from build123d import *

# Parameters (mm, degrees)
F0_W     = 622.3
F0_H     = 530.225
F0_R     = 2.413
F0_R_2   = 4.7625
F0_W_2   = 210.82
F0_H_2   = 310.388
F1_DEPTH = 25.4
F2_T     = -2.54
F3_W     = 617.22
F3_H     = 22.86
F4_DEPTH = 525.145


with BuildPart() as f1:
    # F0 (on Front) → F1 (new body)
    with BuildSketch(Plane.XZ):
        with Locations((0, 265.1125)):
            Rectangle(F0_W, F0_H)
        with Locations((-190.5, 54.483)):
            Circle(F0_R, mode=Mode.SUBTRACT)
        with Locations((-292.1, 95.25)):
            Circle(F0_R_2, mode=Mode.SUBTRACT)
        with Locations((-259.588, 91.694)):
            Circle(F0_R, mode=Mode.SUBTRACT)
        with Locations((-88.9, 54.483)):
            Circle(F0_R, mode=Mode.SUBTRACT)
        with Locations((-19.812, 91.694)):
            Circle(F0_R, mode=Mode.SUBTRACT)
        with Locations((-259.588, 174.244)):
            Circle(F0_R, mode=Mode.SUBTRACT)
        with Locations((-19.812, 174.244)):
            Circle(F0_R, mode=Mode.SUBTRACT)
        with Locations((-139.7, 225.044)):
            Rectangle(F0_W_2, F0_H_2, mode=Mode.SUBTRACT)
        with Locations((88.9, 54.483)):
            Circle(F0_R, mode=Mode.SUBTRACT)
        with Locations((19.812, 91.694)):
            Circle(F0_R, mode=Mode.SUBTRACT)
        with Locations((190.5, 54.483)):
            Circle(F0_R, mode=Mode.SUBTRACT)
        with Locations((259.588, 91.694)):
            Circle(F0_R, mode=Mode.SUBTRACT)
        with Locations((292.1, 95.25)):
            Circle(F0_R_2, mode=Mode.SUBTRACT)
        with Locations((19.812, 174.244)):
            Circle(F0_R, mode=Mode.SUBTRACT)
        with Locations((139.7, 225.044)):
            Rectangle(F0_W_2, F0_H_2, mode=Mode.SUBTRACT)
        with Locations((259.588, 174.244)):
            Circle(F0_R, mode=Mode.SUBTRACT)
        with Locations((-259.588, 275.844)):
            Circle(F0_R, mode=Mode.SUBTRACT)
        with Locations((-259.588, 358.394)):
            Circle(F0_R, mode=Mode.SUBTRACT)
        with Locations((-190.5, 395.605)):
            Circle(F0_R, mode=Mode.SUBTRACT)
        with Locations((-19.812, 275.844)):
            Circle(F0_R, mode=Mode.SUBTRACT)
        with Locations((-88.9, 395.605)):
            Circle(F0_R, mode=Mode.SUBTRACT)
        with Locations((-19.812, 358.394)):
            Circle(F0_R, mode=Mode.SUBTRACT)
        with Locations((-292.1, 476.25)):
            Circle(F0_R_2, mode=Mode.SUBTRACT)
        with Locations((19.812, 275.844)):
            Circle(F0_R, mode=Mode.SUBTRACT)
        with Locations((19.812, 358.394)):
            Circle(F0_R, mode=Mode.SUBTRACT)
        with Locations((88.9, 395.605)):
            Circle(F0_R, mode=Mode.SUBTRACT)
        with Locations((259.588, 275.844)):
            Circle(F0_R, mode=Mode.SUBTRACT)
        with Locations((190.5, 395.605)):
            Circle(F0_R, mode=Mode.SUBTRACT)
        with Locations((259.588, 358.394)):
            Circle(F0_R, mode=Mode.SUBTRACT)
        with Locations((292.1, 476.25)):
            Circle(F0_R_2, mode=Mode.SUBTRACT)
    extrude(amount=F1_DEPTH)

    # F2
    f2_openings = [f1.faces().sort_by_distance(p)[0] for p in [
        (0, 0, 291.607125),
    ]]
    offset(amount=F2_T, openings=f2_openings, kind=Kind.INTERSECTION)

    # F3 (on face) → F4 (cut, through all)
    with BuildSketch(Plane(origin=(0, 0, 527.685), x_dir=(1, 0, 0), z_dir=(0, 0, -1))):
        with Locations((0, 11.43)):
            Rectangle(F3_W, F3_H)
    extrude(amount=F4_DEPTH, mode=Mode.SUBTRACT)


solid = f1.part
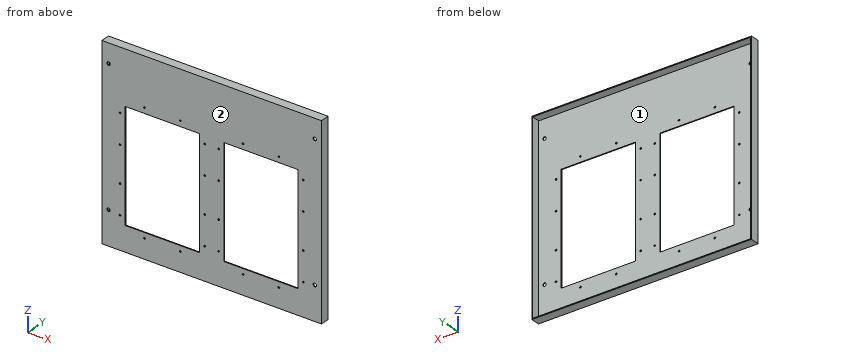
Work out the finished part from the listing and answer in its coordinate system (mm). Face numbers are marked on the shaded views. Give positions to 0.01 mm unless a question says otherwise; leave off trailing zeros. Order: outer loops, then holes, each group sorted by start corner. A loop starts at its lowest first (then second) coordinate and runs counter-clockwise, first axis right, second up. Notation, with made-up numbers: (47.25, 33) -> (95.25, 33) arc R21 cw to (95.25, 51) -> close; hole circle Ø10 at (34, 1.25). An arc over 180 degrees is marked (long way). Answer as a JSON object with one key per item and string values. Group by question number.
1. Section B-B on y = -8 is taken. Determine the outline of the cut face in (x, z) (3 decimals), plus the area to 3 significant figures.
2. Section A-A on x = -60 is taken. Determine the outline of the cut face in (y, z) (3 decimals), plus the area to 3 significant figures.
3. Section C-C on z = 454 is taken. Determine the outline of the cut face in (x, y), plus the area to 3 significant figures.
4. A flat-ended cylindrical pin translates along its axis: pin 1 Ø5.5 at (x, z) = (259.588, 275.844) entering from +Y. Find the tip coordinate at first contact, or state that the pin passes through.
5. The mould has two halves that part along X. Classify the marked faces 1 and 2: released by +X, released by -X, zero draft, split by the parting line, or undercut.
6. Consider line 1 along Z through (x, y) = (-292.1, -24.25) (1 decimal); line 2 along Z through (x, y) = (-190.5, -23.5) (3 decimals); line 3 along X through (y, z) = (-23.65, 476.25). Determine where each line is inside the solid, lowest interval first. Write a range as [from, to].
Result sheet:
{
 "1": {"outline": "(-311.15, 0) -> (311.15, 0) -> (311.15, 530.225) -> (-311.15, 530.225) -> close; hole (-308.61, 2.54) -> (308.61, 2.54) -> (308.61, 527.685) -> (-308.61, 527.685) -> close", "area": "5,830 mm^2"},
 "2": {"outline": "(-25.4, 0) -> (0, 0) -> (0, 2.54) -> (-22.86, 2.54) -> (-22.86, 69.85) -> (-25.4, 69.85) -> close; (-25.4, 380.238) -> (-22.86, 380.238) -> (-22.86, 527.685) -> (0, 527.685) -> (0, 530.225) -> (-25.4, 530.225) -> close", "area": "675 mm^2"},
 "3": {"outline": "(-311.15, -25.4) -> (311.15, -25.4) -> (311.15, 0) -> (308.61, 0) -> (308.61, -22.86) -> (-308.61, -22.86) -> (-308.61, 0) -> (-311.15, 0) -> close", "area": "1,700 mm^2"},
 "4": {"pin 1": "stops at y = -22.86"},
 "5": {"face 1": "undercut", "face 2": "zero draft"},
 "6": {"line 1": "z = [0, 90.5], [100, 471.5], [481, 530.2]", "line 2": "z = [0, 52.07], [56.896, 69.85], [380.238, 393.192], [398.018, 530.225]", "line 3": "x = [-311.15, -296.86], [-287.34, 287.34], [296.86, 311.15]"}
}
